```python
from build123d import *

# Parameters (mm, degrees)
SKETCH1_R           = 6.35
EXTRUDE1_DEPTH      = 152.4
CHAMFER1_SIZE       = 0.9525
SKETCH3_W           = 3.175
SKETCH3_H           = 1.5875
EXTRUDE2_DEPTH      = 153.4
EXTRUDE2_DEPTH_BACK = 153.4


with BuildPart() as part:
    # Sketch1 → Extrude1 (new body, symmetric)
    with BuildSketch(Plane.XY):
        Circle(SKETCH1_R)
    extrude(amount=EXTRUDE1_DEPTH, both=True)

    # Chamfer1
    chamfer1_edges = [part.edges().sort_by_distance(p)[0] for p in [
        (-6.35, 0, -152.4),
        (-6.35, 0, 152.4),
    ]]
    chamfer(chamfer1_edges, length=CHAMFER1_SIZE)

    # Sketch3 → Extrude2 (cut, two sides)
    with BuildSketch(Plane.XY) as extrude2_sk:
        with Locations((0, 5.55625)):
            Rectangle(SKETCH3_W, SKETCH3_H)
    extrude(amount=EXTRUDE2_DEPTH, mode=Mode.SUBTRACT)
    extrude(extrude2_sk.sketch, amount=-EXTRUDE2_DEPTH_BACK, mode=Mode.SUBTRACT)


solid = part.part
```
Read the model definition and answer for the solid it produces. Units are mm, in the model's axes. Coordinates: 2 decimals unless noted, no trailing zeros. Write each loop counter-clockwise with the first axis right and the second up, starting at its lowest first coordinate (ties: lowest second). Pieces come first, ordered by that corner, then holes. Notation, with made-up numbers: (78, 58.25) - (108, 58.25) arc R21 ccw to (108, 69.25) - close; hole circle Ø9 at (70.25, 74). An arc over 180 degrees is marked (long way). Answer as a JSON object with one key per item and string values. Group by question number.
1. The mould has two halves that part along X. Classify faces 1 (the cylindrical face through (-0.257, -6.345, 2.12)), 2 (the flat face through (0, 0, 152.4)): +X half, -X half, draft (parallel to the pull), parting line (faces both ways), or undercut.
2. Consider L1, parallel to Y at x = 0.5, z = 126; L2, parallel to X at y = -0.5, z = 93; L3, parallel to X at y = 5.25, z = 93.5. Determine where each line is inside the solid, lowest interval first. Write a range as [from, to].
3. A cutting plane is placed at A-A (z = -54). Determine the outline of the cut face in (x, y), plus the area to 3 significant figures.
4. Each of these flat-tipped pins is pushed along its axis until it touches: P1, Ø6, axis at x = -1.5, z = -62.5, coming from the -Y side; P2, Ø1, axis at x = -0.5, z = 119.5, coming from the +Y side; P3, Ø1.5, axis at x = 3.5, z = -20, coming from the -Y side; P4, Ø1.1, axis at y = 5.5, z = -67.5, coming from the +X side. Where does it stop, or does it pass through?
Worked out:
{
 "1": {"face 1": "parting line", "face 2": "draft"},
 "2": {"L1": "y = [-6.33, 4.76]", "L2": "x = [-6.33, 6.33]", "L3": "x = [-3.57, -1.59], [1.59, 3.57]"},
 "3": {"outline": "(-1.59, 4.76) - (-1.59, 6.15) arc R6.35 ccw (long way) to (1.59, 6.15) - (1.59, 4.76) - close", "area": "122 mm²"},
 "4": {"P1": "stops at y = -6.35", "P2": "stops at y = 4.76", "P3": "stops at y = -5.72", "P4": "stops at x = 3.98"}
}
